Input: part model. Units: mm. Frame: model coordinates. A direction names the side the tool comes from. Round coordinates to 2 decimals unless told otherwise and drop trailing zeros. Loops run counter-clockwise (first coordinate to the right, second up) from the corner with the lowest first, then second, coordinate; pieces in that order, holes last.
1) Section D-D, the plane z = 13.5. Return loops of the section in (x, y), and give its area (3 significant figures).
2) Access query for faces 1 (the face through (-27.472, -15.052, 4.472)), 2 (the face through (-28.297, -28.359, 9.38)), 3 (the face through (1, 16, 10)). Directions: +Z, -Z, +X, -X, +Y, -Y. A direction counts if a zero-diameter tool reaches every point of the face in a straight line with its end or side. Return the directions, or none.
3) Section B-B, the plane x = 18. Return loops of the section in (y, z), and give its area (4 significant figures).
4) Ray query, line 1 along Y through (x, z) = (6.5, 5.5); line 2 along Y through (x, z) = (-5, 16.75). Return the intervals inside material, ascending.
5) Draft query along Z for faces 4 (the face through (-27, -18, 10.5)), 5 (the face through (1, 12.5, 6)), 6 (the face through (0, -28, 18.5)). Return one class per face: pulls with the +Z half, pulls with the -Z half, needs draft (parallel to the pull), parting line crosses it, or undercut.
6) Section A-A, the plane z = 4.75. Return loops of the section in (x, y), and give its area (3 significant figures).
from build123d import *

# Parameters (mm, degrees)
F0_W      = 59
F0_H      = 59
F0_W_2    = 51
F0_H_2    = 51
F1_DEPTH  = 16
F2_W      = 59
F2_H      = 59
F2_W_2    = 55
F2_H_2    = 55
F3_DEPTH  = 2.5
F4_W      = 51
F4_H      = 51
F5_DEPTH  = 2.5
F7_W      = 2.5
F7_H      = 7
F8_DEPTH  = 10
F9_R      = 0.4
F10_DEPTH = 2.5
F10_TAPER = 0.25
F11_R     = 4
F12_R     = 4
F14_DEPTH = 25


with BuildPart() as f1:
    # F0 (on Top) → F1 (new body)
    with BuildSketch(Plane.XY):
        Rectangle(F0_W, F0_H)
        Rectangle(F0_W_2, F0_H_2, mode=Mode.SUBTRACT)
    extrude(amount=F1_DEPTH)

    # F2 (on face) → F3 (join)
    with BuildSketch(Plane.XY.offset(16)):
        Rectangle(F2_W, F2_H)
        Rectangle(F2_W_2, F2_H_2, mode=Mode.SUBTRACT)
    extrude(amount=F3_DEPTH)

    # F4 (on face) → F5 (join)
    with BuildSketch(Plane(origin=(0, 0, 0), x_dir=(1, 0, 0), z_dir=(0, 0, -1))):
        Rectangle(F4_W, F4_H)
    extrude(amount=-F5_DEPTH)

    # F7 (on face) → F8 (join)
    with BuildSketch(Plane.XY):
        with Locations((1.25, 16)):
            Rectangle(F7_W, F7_H)
    extrude(amount=F8_DEPTH)

    # F9 (on face) → F10 (cut)
    with BuildSketch(Plane(origin=(0, 0, 0), x_dir=(0, -1, 0), z_dir=(-1, 0, 0))):
        with Locations((-17.75, 7.5)):
            Circle(F9_R)
        with Locations((-14.25, 7.5)):
            Circle(F9_R)
    extrude(amount=-F10_DEPTH, taper=F10_TAPER, mode=Mode.SUBTRACT)

    # F11
    f11_edges = [f1.edges().sort_by_distance(p)[0] for p in [
        (29.5, 29.5, 9.25),
    ]]
    fillet(f11_edges, radius=F11_R)

    # F12
    f12_edges = [f1.edges().sort_by_distance(p)[0] for p in [
        (-29.5, 29.5, 9.25),
        (-29.5, -29.5, 9.25),
        (29.5, -29.5, 9.25),
    ]]
    fillet(f12_edges, radius=F12_R)

    # F13 (on face) → F14 (cut)
    with BuildSketch(Plane.YZ.offset(-25.5)):
        Polygon((-16.1905989232, 2.5), (-13.8811978465, 6.5), (-16.1905989232, 10.5), (-20.8094010768, 10.5), (-23.1188021535, 6.5), (-20.8094010768, 2.5), align=None)
    extrude(amount=-F14_DEPTH, mode=Mode.SUBTRACT)


solid = f1.part
Final values:
1. outline: (-29.5, -25.5) arc R4 ccw to (-25.5, -29.5) - (25.5, -29.5) arc R4 ccw to (29.5, -25.5) - (29.5, 25.5) arc R4 ccw to (25.5, 29.5) - (-25.5, 29.5) arc R4 ccw to (-29.5, 25.5) - close; hole (-25.5, -25.5) - (25.5, -25.5) - (25.5, 25.5) - (-25.5, 25.5) - close
1. area: 866 mm2
2. face 1: -X
2. face 2: +Z, -Z, -X, -Y
2. face 3: +Z
3. outline: (-29.5, 0) - (29.5, 0) - (29.5, 18.5) - (27.5, 18.5) - (27.5, 16) - (25.5, 16) - (25.5, 2.5) - (-25.5, 2.5) - (-25.5, 16) - (-27.5, 16) - (-27.5, 18.5) - (-29.5, 18.5) - close
3. area: 265.5 mm2
4. line 1: y = -29.5 to -25.5, 25.5 to 29.5
4. line 2: y = -29.5 to -27.5, 27.5 to 29.5
5. face 4: undercut
5. face 5: needs draft
5. face 6: pulls with the +Z half
6. outline: (-29.5, -25.5) arc R4 ccw to (-25.5, -29.5) - (25.5, -29.5) arc R4 ccw to (29.5, -25.5) - (29.5, 25.5) arc R4 ccw to (25.5, 29.5) - (-25.5, 29.5) arc R4 ccw to (-29.5, 25.5) - (-29.5, -14.89) - (-25.5, -14.89) - (-25.5, 25.5) - (25.5, 25.5) - (25.5, -25.5) - (-25.5, -25.5) - (-25.5, -22.11) - (-29.5, -22.11) - close; (0, 12.5) - (2.5, 12.5) - (2.5, 19.5) - (0, 19.5) - close
6. area: 855 mm2
